Verification items for this drawing (mm, ordinates from the low corner). A direction names the side the tool comes from. Round coordinates to 2 decimals unless told otherwise and drop trailing zeros. Loops run counter-clockwise (first coordinate to the right, second up) from the corner with the lowest first, then second, coordinate; pieces in that order, holes last. Notation, with made-up numbers: M 37,-22.5 L 88,-22.5 A4 ccw 88,-15.5 Z; hole C 87.25,-32.5 d1. An arc over 180 degrees is marked long. Write item = value, one per line. Start each with the question number.
(1) Cross-section at D-D on y = 26. Record the boundary of the cut face in (x, z).
(2) Cross-section at A-A on y = 30.5. Record the boundary of the cut face in (x, z) (3 decimals), plus the area to 3 significant figures.
(3) Go/stop test with flat-tipped pins: P1, Ø1.3, axis at x = 6, y = 11, coming from the +Z side; P2, Ø6, axis at x = 1.5, z = 13, coming from the +Y side; P3, Ø1.5, axis at x = 4, y = 29.5, coming from the +Z side; P4, Ø5.5, axis at x = 4.5, y = 3.5, coming from the -Z side. Record where each tip stops, or that it passes through.
(4) Cross-section at C-C on y = 11. Record the boundary of the cut face in (x, z) (3 decimals), plus the area to 3 significant figures.
(5) Set-up check for the marked faces 1, 2 and 3: record each of +Z, -Z, +X, -X, +Y, -Y from which the full face is reachable in a straight line by a thin tool's end or side.
(6) Scan lines: L1, parallel to X at y = 30.5, z = 18.35 (3 decimals); L2, parallel to X at y = 11, z = 29 (3 decimals); L3, parallel to Z at x = 11.5, y = 27. Record each from-to range of solid material in increasing order. Write a range as from..to.
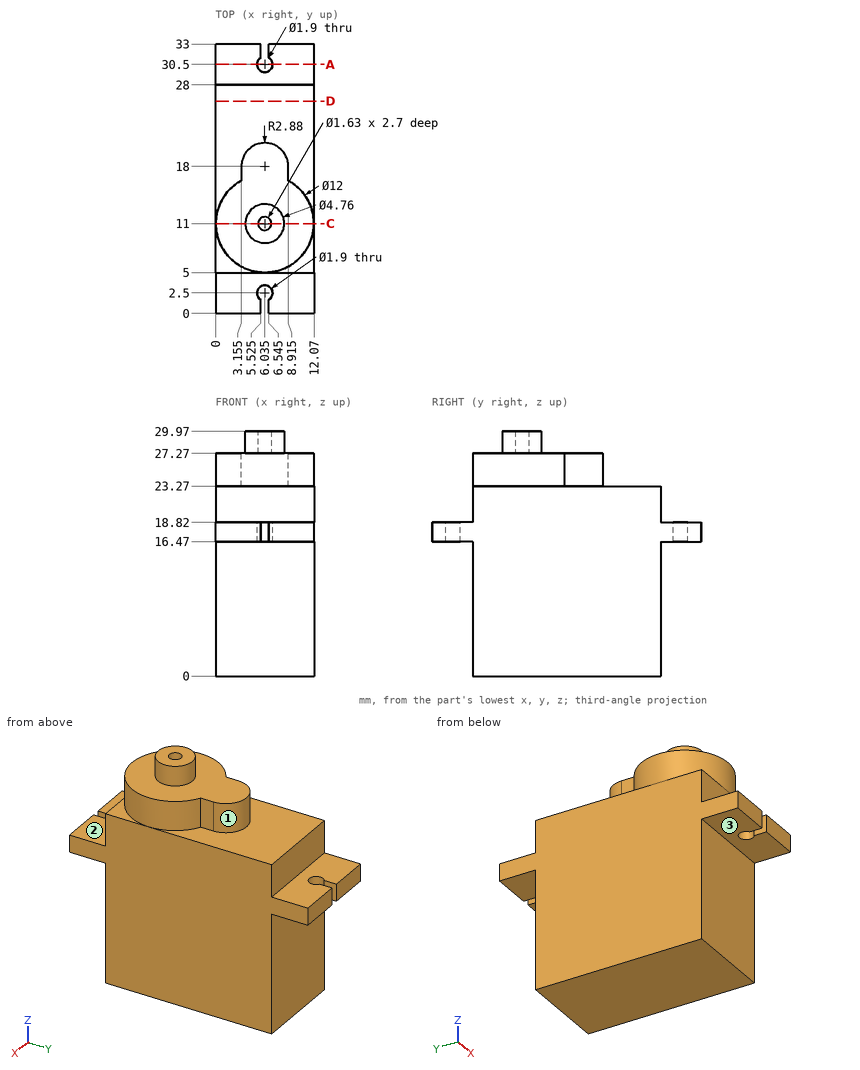
Result:
q1.outline = M 0,0 L 12.07,0 L 12.07,23.27 L 0,23.27 Z
q2.outline = M 0,16.47 L 5.085,16.47 L 5.085,18.82 L 0,18.82 Z; M 6.985,16.47 L 12.07,16.47 L 12.07,18.82 L 6.985,18.82 Z
q2.area = 23.9 mm^2
q3.P1 = 27.27
q3.P2 = 28
q3.P3 = 18.82
q3.P4 = 0
q4.outline = M 0,0 L 12.07,0 L 12.07,23.27 L 12.035,23.27 L 12.035,27.27 L 8.415,27.27 L 8.415,29.97 L 6.85,29.97 L 6.85,27.27 L 5.22,27.27 L 5.22,29.97 L 3.655,29.97 L 3.655,27.27 L 0.035,27.27 L 0.035,23.27 L 0,23.27 Z
q4.area = 337 mm^2
q5.face_1 = +Z, +Y
q5.face_2 = +Z, +X, -X, -Y
q5.face_3 = -Z, +X, -X, -Y
q6.L1 = 0..5.085, 6.985..12.07
q6.L2 = 3.655..5.22, 6.85..8.415
q6.L3 = 0..23.27
